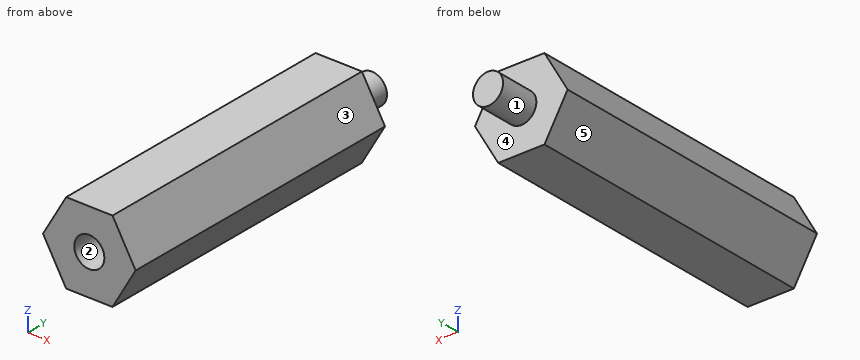
```python
from build123d import *

# Parameters (mm, degrees)
EXTRUDE_1_DEPTH     = 60
SKETCH_2_R          = 3
EXTRUDE_2_DEPTH     = 8
SKETCH_3_R          = 3
CUT_EXTRUDE_1_DEPTH = 8


with BuildPart() as part:
    # 草图1 → 凸台-拉伸1 (new body)
    with BuildSketch(Plane(origin=(0, 0, 0), x_dir=(1, 0, 0), z_dir=(0, 1, 0))):
        Polygon((4.610693432, 8.004676097), (-4.626906133, 7.995315689), (-9.237599565, -0.009360407), (-4.610693432, -8.004676097), (4.626906133, -7.995315689), (9.237599565, 0.009360407), align=None)
    extrude(amount=EXTRUDE_1_DEPTH)

    # 草图2 → 凸台-拉伸2 (add)
    with BuildSketch(Plane(origin=(0, 60, 0), x_dir=(1, 0, 0), z_dir=(0, 1, 0))):
        Circle(SKETCH_2_R)
    extrude(amount=EXTRUDE_2_DEPTH)

    # 草图3 → 切除-拉伸1 (cut)
    with BuildSketch(Plane.XZ):
        Circle(SKETCH_3_R)
    extrude(amount=-CUT_EXTRUDE_1_DEPTH, mode=Mode.SUBTRACT)


solid = part.part
```
The listing builds one solid part. Answer for the finished solid, in the listing's coordinates (mm). Face numbers are marked on the shaded views. A direction names the side the tool comes from. Give positions to 0.01 mm unless a question says otherwise; leave off trailing zeros. Order: outer loops, then holes, each group sorted by start corner. A loop starts at its lowest first (then second) coordinate and runs counter-clockwise, first axis right, second up.
1) Find section C-C on x = -0.5. Write down the section's boundary in (y, z).
Reported:
outline: (0, -8) - (60, -8) - (60, -2.96) - (68, -2.96) - (68, 2.96) - (60, 2.96) - (60, 8) - (0, 8) - (0, 2.96) - (8, 2.96) - (8, -2.96) - (0, -2.96) - close
2) Given P1, Ø6, axis at y = 17.5, z = 3.5, coming from the -X side; P2, Ø3, axis at x = -1, z = 0, coming from the -Y side; P3, Ø2, axis at y = 37, z = 2.5, coming from the +X side, each flat-ended and moving along its own axis, determine where each tip first touches the part or whether it passes through.
Reported:
P1: stops at x = -8.95
P2: stops at y = 8
P3: stops at x = 8.37
3) Find section A-A on z = 1.5. Write down the section's boundary in (x, y), then the cut area to 3 significant figures.
Reported:
outline: (-8.37, 0) - (-2.6, 0) - (-2.6, 8) - (2.6, 8) - (2.6, 0) - (8.37, 0) - (8.37, 60) - (2.6, 60) - (2.6, 68) - (-2.6, 68) - (-2.6, 60) - (-8.37, 60) - close
area: 1,000 mm2
4) Find section D-D on z = 4.75. Write down the section's boundary in (x, y).
Reported:
outline: (-6.49, 0) - (6.5, 0) - (6.5, 60) - (-6.49, 60) - close
5) Consider line 1 along Z through (x, y) = (0, 4); line 2 along Y through (x, z) = (-1.25, -5.75); line 3 along Z through (x, y) = (1.75, 5). Determine where each line is inside the solid, lowest interval first.
Reported:
line 1: z = -8 to -3, 3 to 8
line 2: y = 0 to 60
line 3: z = -8 to -2.44, 2.44 to 8
6) For the marked faces 4 and 5, determine the directions among +Z, -Z, +X, -X, +Y, -Y from which every point of the face is accessible in a straight line to the end or side of a thin tool.
Reported:
face 4: +Y
face 5: -Z, -X, +Y, -Y
7) Determine the mould class of the marked faces 1, 2 and 3 for opening direction Z: pulls with the +Z half, pulls with the -Z half, needs draft (parallel to the pull), parting line crosses it, or undercut.
Reported:
face 1: parting line crosses it
face 2: undercut
face 3: pulls with the +Z half
8) Find section B-B on y = 44.5. Write down the section's boundary in (x, z), then the cut area to 3 significant figures.
Reported:
outline: (-9.24, 0.01) - (-4.63, -8) - (4.61, -8) - (9.24, -0.01) - (4.63, 8) - (-4.61, 8) - close
area: 222 mm2
